from build123d import *

# Parameters (mm, degrees)
SKETCH_1_W          = 41
SKETCH_1_H          = 10
EXTRUDE_1_DEPTH     = 6
SKETCH_2_R          = 0.8
CUT_EXTRUDE_1_DEPTH = 6
FILLET_1_R          = 2
SKETCH_6_R          = 0.8
CUT_EXTRUDE_3_DEPTH = 10


with BuildPart() as part:
    # 草图1 → 凸台-拉伸1 (new body)
    with BuildSketch(Plane(origin=(0, 0, 0), x_dir=(1, 0, 0), z_dir=(0, 1, 0))):
        with Locations((-20.5, 5)):
            Rectangle(SKETCH_1_W, SKETCH_1_H)
    extrude(amount=EXTRUDE_1_DEPTH)

    # 草图2 → 切除-拉伸1 (cut)
    with BuildSketch(Plane.XY):
        with Locations((-6, 3)):
            Circle(SKETCH_2_R)
        with Locations((-35, 3)):
            Circle(SKETCH_2_R)
    extrude(amount=-CUT_EXTRUDE_1_DEPTH, mode=Mode.SUBTRACT)

    # 圆角1
    fillet_1_edges = [part.edges().sort_by_distance(p)[0] for p in [
        (-41, 3, -10),
        (0, 3, -10),
    ]]
    fillet(fillet_1_edges, radius=FILLET_1_R)

    # 草图6 → 切除-拉伸3 (cut)
    with BuildSketch(Plane(origin=(0, 0, 0), x_dir=(-1, 0, 0), z_dir=(0, -1, 0))):
        with Locations(Location((38.5, 4, 0), (0, 0, 90))):
            Circle(SKETCH_6_R)
        with Locations(Location((18, 4, 0), (0, 0, 90))):
            Circle(SKETCH_6_R)
    extrude(amount=-CUT_EXTRUDE_3_DEPTH, mode=Mode.SUBTRACT)


solid = part.part
Geometry check sheet. Reference: the model listing, model coordinates, mm. A direction names the side the tool comes from. Give positions to 0.01 mm unless a question says otherwise; leave off trailing zeros. Loops run counter-clockwise (first coordinate to the right, second up) from the corner with the lowest first, then second, coordinate; pieces in that order, holes last. Notation, with made-up numbers: M 4.25,-5.75 L 26.25,-5.75 A23 cw 26.25,15.25 Z; hole C -10.75,48.25 d11. An arc over 180 degrees is marked long. Answer as a JSON object with one key per item and string values. Group by question number.
Item 1: Sectioned sample at B-B on y = 3. Record the boundary of the cut face in (x, z), plus the area to 3 significant figures.
Item 2: Sectioned sample at D-D on x = -6. Record the boundary of the cut face in (y, z), plus the area to 3 significant figures.
Item 3: Sectioned sample at A-A on z = -4. Record the boundary of the cut face in (x, y), plus the area to 3 significant figures.
Item 4: Sectioned sample at C-C on x = -18. Record the boundary of the cut face in (y, z).
Item 5: Material ranges on L1, parallel to X at y = 4.6, z = -4; L2, parallel to Z at x = -38.5, y = 3.45; L3, parallel to Y at x = -6, z = -3.25, recorded low to high.
Item 6: Access from +Z, -Z, +X, -X, +Y, -Y to the whole of each face (thin tool, end or side, straight path). Record for faces 1 (the flat face through (-41, 3, -4)), 2 (the flat face through (-35, 3, -6)).
Item 7: Mould release check, pull along X, two halves, no side actions. Record for faces 3 (the flat face through (-6, 3, -6)), 4 (the flat face through (0, 3, -4)), 5 (the flat face through (-21, 3, 0)), 6 (the cylindrical face through (-34.237, 3.24, -2.958)): pulls with the +X half, pulls with the -X half, needs draft (parallel to the pull), parting line crosses it, or undercut.
Item 8: Gauge pin test, flat end, axial feed: pin 1 (1.3 mm diameter, centred on x = -35, y = 3, fed in from +Z). Record the tip position at first contact, or that the pin passes through.
Findings below:
{
 "1": {"outline": "M -41,-8 A2 ccw -39,-10 L -2,-10 A2 ccw 0,-8 L 0,0 L -5.2,0 L -5.2,-6 L -6.8,-6 L -6.8,0 L -34.2,0 L -34.2,-6 L -35.8,-6 L -35.8,0 L -41,0 Z; hole C -38.5,-4 d1.6; hole C -18,-4 d1.6", "area": "385 mm2"},
 "2": {"outline": "M 0,-10 L 6,-10 L 6,0 L 3.8,0 L 3.8,-6 L 2.2,-6 L 2.2,0 L 0,0 Z", "area": "50.4 mm2"},
 "3": {"outline": "M -41,0 L -39.3,0 L -39.3,6 L -41,6 Z; M -37.7,0 L -18.8,0 L -18.8,6 L -37.7,6 Z; M -17.2,0 L 0,0 L 0,6 L -17.2,6 Z; hole C -35,3 d1.6; hole C -6,3 d1.6", "area": "223 mm2"},
 "4": {"outline": "M 0,-10 L 6,-10 L 6,-4.8 L 0,-4.8 Z; M 0,-3.2 L 6,-3.2 L 6,0 L 0,0 Z"},
 "5": {"L1": "-41 to -39.3, -37.7 to -18.8, -17.2 to 0", "L2": "-10 to -4.8, -3.2 to 0", "L3": "0 to 2.2, 3.8 to 6"},
 "6": {"face 1": "+Z, -Z, -X, +Y, -Y", "face 2": "+Z"},
 "7": {"face 3": "undercut", "face 4": "pulls with the +X half", "face 5": "needs draft", "face 6": "undercut"},
 "8": {"pin 1": "z = -6"}
}
